Verification items for the finished model (mm, model axes). Face numbers are marked on the shaded views. A direction names the side the tool comes from. Coordinates: 2 decimals unless noted, no trailing zeros. Order: outer loops, then holes, each group sorted by start corner. A loop starts at its lowest first (then second) coordinate and runs counter-clockwise, first axis right, second up.
Q1. Depth check by flat-ended pin: P1, Ø10, axis at x = 7, y = -80.5, coming from the +Z side; P2, Ø1.5, axis at y = 37, z = 2.5, coming from the -X side; P3, Ø3, axis at x = -1.5, y = 8.5, coming from the +Z side. Enter the tip coordinate at first touch or a pass-through.
Q2. Cross-section at B-B, the plane y = -28.5. Record the boundary of the cut face in (x, z), and give its area (3 significant figures).
Q3. Set-up check for the marked faces 3 and 4: record each of +Z, -Z, +X, -X, +Y, -Y from which the full face is reachable in a straight line by a thin tool's end or side.
Q4. Draft check along Z on the marked faces 1 and 2. Enter one of: pulls with the +Z half, pulls with the -Z half, needs draft (parallel to the pull), parting line crosses it, or undercut.
Q5. Cross-section at C-C, the plane y = 11. Record the boundary of the cut face in (x, z), and give its area (3 significant figures).
Q6. Cross-section at A-A, the plane y = 33. Record the boundary of the cut face in (x, z).
Q7. Thickness scan on line 1 (Z direction, x = 0, y = 37.5); line 2 (X direction, y = 65, z = 1.75). Record the ranges inside material, lowest first.
from build123d import *

# Parameters (mm, degrees)
F2_SIZE = 0.5


# Not quite as in the source:
# - a fillet or chamfer that OpenCascade refuses, or shapes differently, is made with other operations: its cross-section is extruded or revolved along the edge and cut away or added


with BuildPart() as f1:
    # F0 (on Right) → F1 (revolve)
    with BuildSketch(Plane.YZ):
        Polygon((103.6051637142, 6), (103.6051637142, 9), (15.6051637142, 9), (-88.3948362864, 5), (-88.3948362864, 7), (-91.3948362864, 7), (-91.3948362864, 5), (-114.3948362864, 5), (-114.3948362864, 0), (0, 0), (3.6051637142, 6), align=None)
    revolve(axis=Axis((0, -57.1974181432, 0), (0, -1, 0)))

    # F2
    f2_edges = [f1.edges().sort_by_distance(p)[0] for p in [
        (0, -91.394836, -7),
        (0, -88.394836, -7),
        (0, -114.394836, -5),
    ]]
    chamfer(f2_edges, length=F2_SIZE)

    # F3: fillet of radius 2 on 1 edges, made by hand

    # F3_s1 → F3_t2 (revolve)
    with BuildSketch(Plane.YZ):
        with BuildLine():
            ThreePointArc((-88.3948362864, 6.5), (-87.641927013, 5.4477782371), (-86.4024545248, 5.0766300678))
            Line((-86.4024545248, 5.0766300678), (-86.4009172, 5.0366596208))
            Line((-86.4009172, 5.0366596208), (-88.3932989615, 4.960029553))
            Line((-88.3932989615, 4.960029553), (-88.4348362864, 5))
            ThreePointArc((-88.4348362864, 5), (-88.4348362864, 5.75), (-88.4331465967, 6.4884969517))
            Line((-88.4331465967, 6.4884969517), (-88.3948362864, 6.5))
        make_face()
    revolve(axis=Axis((0, -88.3948362864, 0), (0, -1, 0)))


solid = f1.part
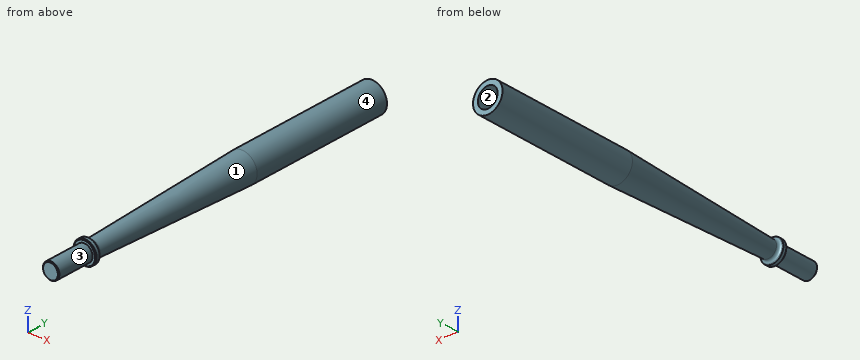
Check values:
1. P1: stops at z = 4.92
1. P2: stops at x = -8.83
1. P3: stops at z = 8.76
2. outline: circle Ø14.61 at (0, 0)
2. area: 168 mm2
3. face 3: -Y
3. face 4: +Y, -Y
4. face 1: parting line crosses it
4. face 2: undercut
5. outline: circle Ø17.65 at (0, 0); hole circle Ø12 at (0, 0)
5. area: 131 mm2
6. outline: circle Ø18 at (0, 0); hole circle Ø12 at (0, 0)
7. line 1: z = -9 to -6, 6 to 9
7. line 2: x = -8.83 to -5.74, 5.74 to 8.83
